from build123d import *

# Parameters (mm, degrees)
SKETCH1_W                      = 100
SKETCH1_H                      = 337
SKETCH1_R                      = 17
SKETCH1_R_2                    = 2.5
SKETCH1_R_3                    = 2
BOSS_EXTRUDE1_DEPTH            = 20
CHAMFER1_SIZE                  = 45
SKETCH2_W                      = 100
SKETCH2_H                      = 34
CUT_EXTRUDE1_DEPTH             = 5
CBORE_FOR_M4_SHCS1_D           = 4.5
CBORE_FOR_M4_SHCS1_CBORE_D     = 8
CBORE_FOR_M4_SHCS1_CBORE_DEPTH = 4
CBORE_FOR_M4_SHCS2_D           = 4.5
CBORE_FOR_M4_SHCS2_CBORE_D     = 8
CBORE_FOR_M4_SHCS2_CBORE_DEPTH = 4
M4_TAPPED_HOLE1_D              = 3.3
M4_TAPPED_HOLE1_DEPTH          = 16.1
M4_TAPPED_HOLE1_TIP            = 0.991420021
M4_TAPPED_HOLE2_D              = 3.3


with BuildPart() as part:
    # Sketch1 → Boss-Extrude1 (new body)
    with BuildSketch(Plane.XY):
        with Locations((47.704546062, 452.000370419)):
            Rectangle(SKETCH1_W, SKETCH1_H)
        with Locations((65.704546062, 560.500370419)):
            Circle(SKETCH1_R, mode=Mode.SUBTRACT)
        with Locations((80.553788467, 575.349612824)):
            Circle(SKETCH1_R_2, mode=Mode.SUBTRACT)
        with Locations((80.553788467, 545.651128014)):
            Circle(SKETCH1_R_2, mode=Mode.SUBTRACT)
        with Locations((50.855303657, 545.651128014)):
            Circle(SKETCH1_R_2, mode=Mode.SUBTRACT)
        with Locations((50.855303657, 575.349612824)):
            Circle(SKETCH1_R_2, mode=Mode.SUBTRACT)
        with Locations((34.704546062, 358.500370419)):
            Circle(SKETCH1_R_3, mode=Mode.SUBTRACT)
        with Locations((60.704546062, 358.500370419)):
            Circle(SKETCH1_R_3, mode=Mode.SUBTRACT)
        with Locations((34.704546062, 332.500370419)):
            Circle(SKETCH1_R_3, mode=Mode.SUBTRACT)
        with Locations((60.704546062, 332.500370419)):
            Circle(SKETCH1_R_3, mode=Mode.SUBTRACT)
    extrude(amount=BOSS_EXTRUDE1_DEPTH)

    # Chamfer1
    chamfer1_edges = [part.edges().sort_by_distance(p)[0] for p in [
        (-2.295453938, 620.500370419, 10),
    ]]
    chamfer(chamfer1_edges, length=CHAMFER1_SIZE)

    # Sketch2 → Cut-Extrude1 (cut)
    with BuildSketch(Plane.XY):
        with Locations((47.704546062, 345.500370419)):
            Rectangle(SKETCH2_W, SKETCH2_H)
    extrude(amount=CUT_EXTRUDE1_DEPTH, mode=Mode.SUBTRACT)

    # CBORE for M4 SHCS1 (through all)
    with Locations(Plane.XY.offset(20)):
        with Locations((92.704546062, 610.500370419), (92.704546062, 585.500370419), (92.704546062, 560.500370419), (92.704546062, 535.500370419), (92.704546062, 510.500370419)):
            CounterBoreHole(CBORE_FOR_M4_SHCS1_D / 2, CBORE_FOR_M4_SHCS1_CBORE_D / 2, CBORE_FOR_M4_SHCS1_CBORE_DEPTH)

    # CBORE for M4 SHCS2 (through all)
    with Locations(Plane(origin=(34.704546062, 358.500370419, 20), x_dir=(1, 0, 0), z_dir=(0, 0, 1))):
        with Locations((0, 0), (26, 0), (0, -26), (26, -26)):
            CounterBoreHole(CBORE_FOR_M4_SHCS2_D / 2, CBORE_FOR_M4_SHCS2_CBORE_D / 2, CBORE_FOR_M4_SHCS2_CBORE_DEPTH)

    # M4 Tapped Hole1
    with Locations(Plane(origin=(7.704546062, 283.500370419, 10), x_dir=(0, 0, -1), z_dir=(0, -1, 0))):
        with Locations((0, 0), (0, 20), (0, 60), (0, 80)):
            Hole(M4_TAPPED_HOLE1_D / 2, depth=M4_TAPPED_HOLE1_DEPTH)
            with Locations((0, 0, -(M4_TAPPED_HOLE1_DEPTH + M4_TAPPED_HOLE1_TIP / 2))):  # 118° drill point
                Cone(0, M4_TAPPED_HOLE1_D / 2, M4_TAPPED_HOLE1_TIP, mode=Mode.SUBTRACT)

    # M4 Tapped Hole2 (through all)
    with Locations(Plane.XY.offset(20)):
        with Locations((92.704546062, 566.40602011), (92.704546062, 526.40602011)):
            Hole(M4_TAPPED_HOLE2_D / 2)


solid = part.part
Input: part model. Units: mm. Frame: model coordinates. A direction names the side the tool comes from. Coordinates: 2 decimals unless noted, no trailing zeros.
1. Access query for faces 1 (the cylindrical face through (60.184, 362.466, 18.028)), 2 (the flat face through (47, 346, 5)), 3 (the flat face through (-2.295, 427, 10)). Directions: +Z, -Z, +X, -X, +Y, -Y. A direction counts if a zero-diameter tool reaches every point of the face in a straight line with its end or side. Return the directions, or none.
Checked values:
face 1: +Z
face 2: -Z, +X, -X
face 3: +Z, -Z, -X, +Y, -Y
2. Contact query for flat-ended pins moving along their axis: P1, Ø4, axis at x = 7.7, z = 10, coming from the +Y side; P2, Ø2, axis at x = 29.5, z = 10.5, coming from the +Y side; P3, Ø5, axis at x = 60.7, y = 332.5, coming from the -Z side. Output: stop coordinate, or through.
Checked values:
P1: stops at y = 587.5
P2: stops at y = 608.3
P3: stops at z = 5
3. Draft query along Y for faces 4 (the cylindrical face through (91.837, 556.595, 18.028)), 5 (the flat face through (47, 306, 0)), 6 (the flat face through (70, 620.5, 10)). Return one class per face: +Y half, -Y half, draft (parallel to the pull), parting line (faces both ways), or undercut.
Checked values:
face 4: undercut
face 5: draft
face 6: +Y half
4. Ray query, line 1 along Y through (x, z) = (54, 12.5); line 2 along X through (y, z) = (331, 8.75); line 3 along Y through (x, z) = (33, 7.75). Return the intervals inside material, ascending.
Checked values:
line 1: y = 283.5 to 548.17, 572.83 to 620.5
line 2: x = -2.3 to 33.03, 36.38 to 59.03, 62.38 to 97.7
line 3: y = 283.5 to 331.03, 333.97 to 357.03, 359.97 to 610.8
